The figure shows three views and two pictorial views of one solid part (mm, origin at its lowest corner). Answer the questions. Coordinates: 2 decimals unless noted, no trailing zeros. Loops run counter-clockwise (first coordinate to the right, second up) from the corner with the lowest first, then second, coordinate; pieces in that order, holes last. Notation, with made-up numbers: (46.5, 47.5) - (57.5, 47.5) arc R28 cw to (57.5, 76.5) - close; hole circle Ø6 at (57.25, 59). An arc over 180 degrees is marked (long way). One line per question, with ' | ' between items.
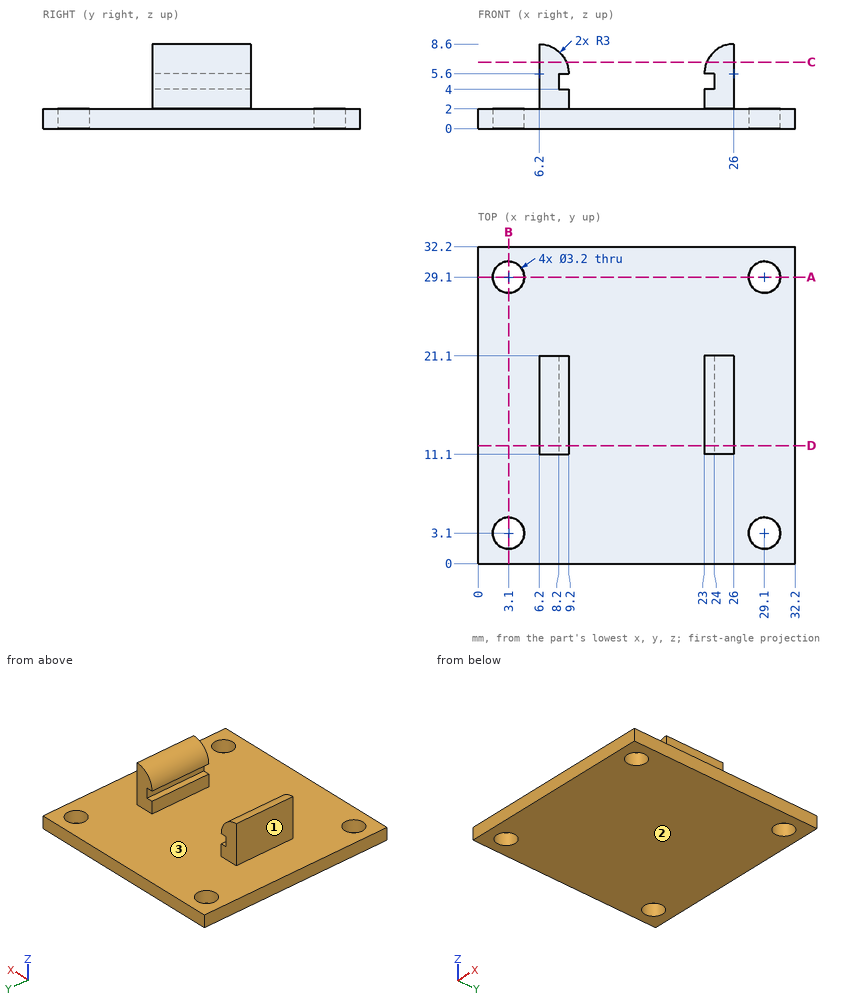
Item 1: The mould has two halves that part along X. Classify the marked faces 1, 2 and 3: pulls with the +X half, pulls with the -X half, needs draft (parallel to the pull), parting line crosses it, or undercut.
Taken from the geometry:
face 1: pulls with the -X half | face 2: needs draft | face 3: undercut
Item 2: Each of these flat-tipped pins is pushed along its axis until it touches: pin 1 Ø3.5 at (x, z) = (8.5, 4.5) entering from +Y; pin 2 Ø1 at (y, z) = (15, 6) entering from +X; pin 3 Ø0.5 at (x, y) = (23.5, 14.5) entering from +Z; pin 4 Ø2.5 at (x, y) = (29.1, 29.1) entering from -Z. Where does it stop, or does it pass through?
Taken from the geometry:
pin 1: stops at y = 21.1 | pin 2: stops at x = 26 | pin 3: stops at z = 7.58 | pin 4: passes through
Item 3: Find section D-D, the plane y = 12. Write down the section's boundary in (x, z), plus the area to 3 significant figures.
Taken from the geometry:
outline: (0, 0) - (32.2, 0) - (32.2, 2) - (26, 2) - (26, 8.6) arc R3 ccw to (23, 5.6) - (24, 5.6) - (24, 4) - (23, 4) - (23, 2) - (9.2, 2) - (9.2, 4) - (8.2, 4) - (8.2, 5.6) - (9.2, 5.6) arc R3 ccw to (6.2, 8.6) - (6.2, 2) - (0, 2) - close | area: 96.9 mm2
Item 4: Find the intervals of material crossed by line 1 (X direction, y = 29.1, z = 1.45); line 2 (X direction, y = 19, z = 2.75), in increasing order. Write a range as [from, to].
Taken from the geometry:
line 1: x = [0, 1.5], [4.7, 27.5], [30.7, 32.2] | line 2: x = [6.2, 9.2], [23, 26]
Item 5: Find section C-C, the plane z = 6.75. Write down the section's boundary in (x, y), plus the area to 3 significant figures.
Taken from the geometry:
outline: (6.2, 11.1) - (8.97, 11.1) - (8.97, 21.1) - (6.2, 21.1) - close; (23.23, 11.1) - (26, 11.1) - (26, 21.1) - (23.23, 21.1) - close | area: 55.4 mm2
Item 6: Find section A-A, the plane y = 29.1. Write down the section's boundary in (x, z), plus the area to 3 significant figures.
Taken from the geometry:
outline: (0, 0) - (1.5, 0) - (1.5, 2) - (0, 2) - close; (4.7, 0) - (27.5, 0) - (27.5, 2) - (4.7, 2) - close; (30.7, 0) - (32.2, 0) - (32.2, 2) - (30.7, 2) - close | area: 51.6 mm2
